Check sheet for the modelled part. Datum: model origin and axes. Units: mm. A direction names the side the tool comes from. Round coordinates to 2 decimals unless told otherwise and drop trailing zeros. Loops run counter-clockwise (first coordinate to the right, second up) from the corner with the lowest first, then second, coordinate; pieces in that order, holes last. Notation, with made-up numbers: (-18.5, 81) -> (-2.5, 81) arc R19 cw to (-2.5, 100) -> close; hole circle Ø5 at (14.25, -10). An arc over 180 degrees is marked (long way). Return JSON: item names as keys, results as strings.
from build123d import *

# Parameters (mm, degrees)
BOX002_W     = 20
BOX002_H     = 30
BOX002_DEPTH = 10
BOX_W        = 7.75
BOX_H        = 7.6
BOX_DEPTH    = 10
BOX001_W     = 20
BOX001_H     = 40
BOX001_DEPTH = 10
FILLET_R     = 0.5


with BuildPart() as cube002:
    # Box002 → Box002 (new body)
    with BuildSketch(Plane(origin=(0, 11, 3), x_dir=(1, 0, 0), z_dir=(0, 0, 1))):
        with Locations((10, 15)):
            Rectangle(BOX002_W, BOX002_H)
    extrude(amount=BOX002_DEPTH)


with BuildPart() as cube:
    # Box → Box (new body)
    with BuildSketch(Plane(origin=(6, 0, 0), x_dir=(1, 0, 0), z_dir=(0, 0, 1))):
        with Locations((3.875, 3.8)):
            Rectangle(BOX_W, BOX_H)
    extrude(amount=BOX_DEPTH)


with BuildPart() as fillet_body:
    # Box001 → Box001 (new body)
    with BuildSketch(Plane.XY):
        with Locations((10, 20)):
            Rectangle(BOX001_W, BOX001_H)
    extrude(amount=BOX001_DEPTH)

    # Cut: cut Cube
    add(cube.part, mode=Mode.SUBTRACT)

    # Cut001: cut Cube002
    add(cube002.part, mode=Mode.SUBTRACT)

    # Fillet
    fillet_edges = [fillet_body.edges().sort_by_distance(p)[0] for p in [
        (0, 5.5, 10),
        (0, 11, 6.5),
        (0, 25.5, 3),
        (0, 40, 1.5),
        (0, 20, 0),
        (0, 0, 5),
        (20, 5.5, 10),
        (16.875, 0, 10),
        (13.75, 3.8, 10),
        (9.875, 7.6, 10),
        (6, 3.8, 10),
        (3, 0, 10),
        (10, 11, 10),
        (20, 11, 6.5),
        (10, 11, 3),
        (10, 40, 3),
        (20, 25.5, 3),
        (20, 40, 1.5),
        (10, 40, 0),
        (20, 20, 0),
        (16.875, 0, 0),
        (13.75, 3.8, 0),
        (9.875, 7.6, 0),
        (6, 3.8, 0),
        (3, 0, 0),
        (6, 0, 5),
        (20, 0, 5),
        (13.75, 0, 5),
    ]]
    fillet(fillet_edges, radius=FILLET_R)


solid = fillet_body.part
Q1. Draft check along X on faces 1 (the flat face through (6, 4, 5)), 2 (the flat face through (10, 20, 0)), 3 (the flat face through (0, 11, 2)). Enter one of: released by +X, released by -X, zero draft, split by the parting line, or undercut.
Results list:
{"face 1": "undercut", "face 2": "zero draft", "face 3": "released by -X"}
Q2. Section check C-C (y = 36.5). Record the boundary of the cut face in (x, z), then the cut area to 3 significant figures.
Results list:
{"outline": "(0, 0.5) arc R0.5 ccw to (0.5, 0) -> (19.5, 0) arc R0.5 ccw to (20, 0.5) -> (20, 2.5) arc R0.5 ccw to (19.5, 3) -> (0.5, 3) arc R0.5 ccw to (0, 2.5) -> close", "area": "59.8 mm^2"}
Q3. Section check B-B (z = 8). Record the boundary of the cut face in (x, y), then the cut area to 3 significant figures.
Results list:
{"outline": "(0, 0.5) arc R0.5 ccw to (0.5, 0) -> (5.5, 0) arc R0.5 ccw to (6, 0.5) -> (6, 7.6) -> (13.75, 7.6) -> (13.75, 0.5) arc R0.5 ccw to (14.25, 0) -> (19.5, 0) arc R0.5 ccw to (20, 0.5) -> (20, 10.5) arc R0.5 ccw to (19.5, 11) -> (0.5, 11) arc R0.5 ccw to (0, 10.5) -> close", "area": "161 mm^2"}
Q4. Material ranges on line 1 (Z direction, x = 3.75, y = 13.5); line 2 (Y direction, x = 12.5, z = 6.25); line 3 (Y direction, x = 19.25, z = 9.25), recorded low to high.
Results list:
{"line 1": "0 to 3", "line 2": "7.6 to 11", "line 3": "0 to 11"}
Q5. Section check A-A (x = 9). Record the boundary of the cut face in (y, z).
Results list:
{"outline": "(7.6, 0.5) arc R0.5 ccw to (8.1, 0) -> (39.5, 0) arc R0.5 ccw to (40, 0.5) -> (40, 2.5) arc R0.5 ccw to (39.5, 3) -> (11.5, 3) arc R0.5 cw to (11, 3.5) -> (11, 9.5) arc R0.5 ccw to (10.5, 10) -> (8.1, 10) arc R0.5 ccw to (7.6, 9.5) -> close"}
Q6. Go/stop test with flat-tipped pins: pin 1 (3 mm diameter, centred on x = 7, z = 7, fed in from +Y); pin 2 (5.5 mm diameter, centred on x = 11.5, y = 27, fed in from +Z); pin 3 (6 mm diameter, centred on y = 31, z = 3.5, fed in from -X); pin 4 (6 mm diameter, centred on x = 10, z = 4, fed in from -Y). Record where each tip stops, or that it passes through.
Results list:
{"pin 1": "y = 11", "pin 2": "z = 3", "pin 3": "x = 0", "pin 4": "y = 7.6"}
Q7. Section check D-D (z = 1.5). Record the boundary of the cut face in (x, y), then the cut area to 3 significant figures.
Results list:
{"outline": "(0, 0.5) arc R0.5 ccw to (0.5, 0) -> (5.5, 0) arc R0.5 ccw to (6, 0.5) -> (6, 7.6) -> (13.75, 7.6) -> (13.75, 0.5) arc R0.5 ccw to (14.25, 0) -> (19.5, 0) arc R0.5 ccw to (20, 0.5) -> (20, 39.5) arc R0.5 ccw to (19.5, 40) -> (0.5, 40) arc R0.5 ccw to (0, 39.5) -> close", "area": "741 mm^2"}
Q8. Tool access check on faces 4 (the flat face through (10, 7.6, 5)), 5 (the flat face through (10, 26, 3)), 6 (the flat face through (3, 0, 5)). Record the directions out of +Z, -Z, +X, -X, +Y, -Y that give a thin tool (end or side, any length) a straight path to the whole face; none if there is none.
Results list:
{"face 4": "+Z, -Z, -Y", "face 5": "+Z, +X, -X, +Y", "face 6": "+Z, -Z, +X, -X, -Y"}
